The model under review builds one solid part; all positions refer to its coordinate system, in mm. A direction names the side the tool comes from. Round coordinates to 2 decimals unless told otherwise and drop trailing zeros. Order: outer loops, then holes, each group sorted by start corner. A loop starts at its lowest first (then second) coordinate and runs counter-clockwise, first axis right, second up.
```python
from build123d import *

# Parameters (mm, degrees)
BOSS_EXTRUDE2_DEPTH         = 22.225
CUT_EXTRUDE2_REACH          = 59.15
SKETCH7_R                   = 7.9375
F_3_8_16_TAPPED_HOLE1_D     = 7.9375
F_3_8_16_TAPPED_HOLE1_DEPTH = 25.4
F_3_8_16_TAPPED_HOLE1_TIP   = 2.384665582


with BuildPart() as part:
    # Sketch1 → Boss-Extrude2 (new body)
    with BuildSketch(Plane(origin=(0, 0, 0), x_dir=(0, 0, -1), z_dir=(1, 0, 0))):
        Polygon((21.525976172, 126.619), (-45.784023828, -19.431), (-45.784023828, -25.781), (30.415976172, -25.781), (30.415976172, 126.619), align=None)
    extrude(amount=BOSS_EXTRUDE2_DEPTH)

    # Sketch4 → CBORE for 3/8 Socket Head Cap Screw1 (revolve, cut)
    with BuildSketch(Plane(origin=(11.1125, 96.139, -11.365976172), x_dir=(0, -1, 0), z_dir=(1, 0, 0))):
        Polygon((0, 0), (0, 19.05), (4.9022, 19.05), (4.9022, 9.525), (7.9375, 9.525), (7.9375, 0), align=None)
    revolve(axis=Axis((11.1125, 96.139, -5.015976172), (0, 0, -1)), mode=Mode.SUBTRACT)

    # Sketch6 → CBORE for 3/8 Socket Head Cap Screw2 (revolve, cut)
    with BuildSketch(Plane(origin=(11.1125, 37.719, -10.095976172), x_dir=(0, -1, 0), z_dir=(1, 0, 0))):
        Polygon((0, 0), (0, 20.32), (4.9022, 20.32), (4.9022, 9.525), (7.9375, 9.525), (7.9375, 0), align=None)
    revolve(axis=Axis((11.1125, 37.719, -3.745976172), (0, 0, -1)), mode=Mode.SUBTRACT)

    # Sketch7 → Cut-Extrude2 (cut, up to next)
    with BuildSketch(Plane(origin=(0, 96.139, -11.365976172), x_dir=(1, 0, 0), z_dir=(0, 0, 1)), mode=Mode.PRIVATE) as cut_extrude2_sk1:
        with Locations((11.1125, -58.42)):
            Circle(SKETCH7_R)
    cut_extrude2_tool1 = extrude(cut_extrude2_sk1.sketch, amount=CUT_EXTRUDE2_REACH, mode=Mode.PRIVATE) & part.part
    add(cut_extrude2_tool1.solids().sort_by_distance((11.1125, 37.719, -11.365976))[0], mode=Mode.SUBTRACT)
    # Sketch7 → Cut-Extrude2 (cut, up to next)
    with BuildSketch(Plane(origin=(0, 96.139, -11.365976172), x_dir=(1, 0, 0), z_dir=(0, 0, 1)), mode=Mode.PRIVATE) as cut_extrude2_sk2:
        with Locations((11.1125, 0)):
            Circle(SKETCH7_R)
    cut_extrude2_tool2 = extrude(cut_extrude2_sk2.sketch, amount=CUT_EXTRUDE2_REACH, mode=Mode.PRIVATE) & part.part
    add(cut_extrude2_tool2.solids().sort_by_distance((11.1125, 96.139, -11.365976))[0], mode=Mode.SUBTRACT)

    # 3/8-16 Tapped Hole1
    with Locations(Plane(origin=(11.1125, -25.781, -15.175976172), x_dir=(0, 0, -1), z_dir=(0, -1, 0))):
        with Locations((0, 0), (-40.64, 0)):
            Hole(F_3_8_16_TAPPED_HOLE1_D / 2, depth=F_3_8_16_TAPPED_HOLE1_DEPTH)
            with Locations((0, 0, -(F_3_8_16_TAPPED_HOLE1_DEPTH + F_3_8_16_TAPPED_HOLE1_TIP / 2))):  # 118° drill point
                Cone(0, F_3_8_16_TAPPED_HOLE1_D / 2, F_3_8_16_TAPPED_HOLE1_TIP, mode=Mode.SUBTRACT)


solid = part.part
```
(1) Consider section B-B (x = 13.5). State how many separate pieces and enclosed holes the cut face has, and give its area (3 significant figures).
Data:
separate pieces: 3
enclosed holes: 0
area: 5,400 mm2
(2) Draft analysis for pull direction Z (two halves, no side actions). For faces 4 (the flat face through (0, 35, 0)), 5 (the cylindrical face through (7.24, -12.9, -16.04)), 6 (the flat face through (7, 100, -20.891)), state which applies: pulls with the +Z half, pulls with the -Z half, needs draft (parallel to the pull), parting line crosses it, or undercut.
Data:
face 4: needs draft
face 5: undercut
face 6: pulls with the +Z half
(3) To check wall thickness, follow probe 1 along Y at (x, z) = (5.75, -14); probe 2 along Z at (x, y) = (7.25, 34.5); probe 3 along Y at (x, z) = (14.5, -8.5). State the ranges of each line that lie inside material, in increasing order.
Data:
probe 1: y = -25.78 to 31.87, 43.57 to 90.29, 101.99 to 110.29
probe 2: z = -30.42 to -19.62
probe 3: y = -25.78 to 30.54, 44.9 to 88.96
(4) For faces 1 (the flat face through (15, 34, -19.621)), 2 (the flat face through (11, 126.619, -26)), 3 (the cylindrical face through (8.698, -12.903, 22.315)), list the 3-axis set-ups (+Z, -Z, +X, -X, +Y, -Y) from which the entire face can be reached by the end or side of a thin tool; tool diameter is ignored.
Data:
face 1: +Z
face 2: +Z, -Z, +X, -X, +Y
face 3: -Y
(5) Insertion check: pin 1 (5 mm diameter, centred on x = 19, y = 104.5, fed in from +Z); pin 2 (11.5 mm diameter, centred on x = 11.11, y = 37.72, fed in from +Z); pin 3 (8 mm diameter, centred on y = 50, z = 16.5, fed in from -X); pin 4 (7 mm diameter, centred on x = 11.11, z = -15.18, fed in from +Y). Each pin has a flat end and moves straight along its axis. Give the tip position at first contact, or say it passes through.
Data:
pin 1: stops at z = -10.18
pin 2: stops at z = -19.62
pin 3: stops at x = 0
pin 4: stops at y = 120.44
(6) Consider section D-D (y = 10). Write out the cut boundary in (x, z) (3 decimals), and give its area (3 significant figures).
Data:
outline: (0, -30.416) - (22.225, -30.416) - (22.225, 32.22) - (0, 32.22) - close
area: 1,390 mm2
